Geometry: final body of the model. Coordinates: model frame, mm. A direction names the side the tool comes from. Round coordinates to 2 decimals unless told otherwise and drop trailing zeros. Order: outer loops, then holes, each group sorted by start corner. A loop starts at its lowest first (then second) coordinate and runs counter-clockwise, first axis right, second up. Notation, with made-up numbers: M 83.5,80 L 113.5,80 A19 cw 113.5,113 Z; hole C 60.5,-37 d7. An arc over 180 degrees is marked long. Put each result on its own line as item: value. Start each with the question number.
1) Section A-A, the plane x = -5. Return loops of the section in (y, z) (3 decimals).
2) Section D-D, the plane x = 9.5. Return loops of the section in (y, z), then the cut area to 3 significant figures.
3) Access query for faces 1 (the flat face through (6.25, 0, 0)), 2 (the flat face through (-25, 0, 0)). Directions: +Z, -Z, +X, -X, +Y, -Y. A direction counts if a zero-diameter tool reaches every point of the face in a straight line with its end or side. Return the directions, or none.
4) First-contact query: P1, Ø3, axis at x = -21.92, z = -21.92, coming from the +Y side. Flat tip, straight axial feed; report the tip coordinate or a pass-through.
5) Section C-C, the plane y = -0.85. Return loops of the section in (x, z) (3 decimals), then the cut area to 3 significant figures.
6) Draft query along X for faces 3 (the flat face through (0, 0, -25)), 4 (the cylindrical face through (23.797, 0.02, 23.859)), 5 (the flat face through (0, 0, -11.625)), 6 (the flat face through (-6.25, 0, 0)). Return one class per face: pulls with the +X half, pulls with the -X half, needs draft (parallel to the pull), parting line crosses it, or undercut.
7) Section B-B, the plane z = 0. Return loops of the section in (x, y).
8) Material intervals for probe 1 along X at (y, z) = (0.6, 0); probe 2 along Z at (x, y) = (2, -0.3) (3 decimals); probe 3 along X at (y, z) = (0.4, -10.5), sorted ascending. Write a range as [from, to].
Autodesk Inventor part; units mm, degrees
ref_plane "YZ Plane" through (0, 0, 0) normal (1, 0, 0) x (0, 1, 0)
ref_plane "XZ Plane" through (0, 0, 0) normal (0, 1, 0) x (-1, 0, 0)
ref_plane "XY Plane" through (0, 0, 0) normal (0, 0, 1) x (1, 0, 0)
sketch "Sketch1" plane through (0, 0, 0) normal (0, 1, 0) x (-1, 0, 0)
  line L0 (-25, 25) -> (25, 25)
  line L1 (25, 25) -> (25, -25)
  line L2 (25, -25) -> (-25, -25)
  line L3 (-25, -25) -> (-25, 25)
  line L4 (-25, 25) -> (25, -25) construction
  line L5 (25, 25) -> (-25, -25) construction
  point P0 (0, 0)
  dimension "d0" = 50
extrude "Extrusion1" add sketch "Sketch1" along normal mid plane 2.8
sketch "Sketch2" plane through (0, 1.4, 0) normal (0, 1, 0) x (1, 0, 0)
  line L0 (-6.25, -11.625) -> (6.25, -11.625)
  line L1 (6.25, -11.625) -> (6.25, 11.625)
  line L2 (6.25, 11.625) -> (-6.25, 11.625)
  line L3 (-6.25, 11.625) -> (-6.25, -11.625)
  line L4 (-6.25, -11.625) -> (6.25, 11.625) construction
  line L5 (6.25, -11.625) -> (-6.25, 11.625) construction
  point P0 (0, 0)
  dimension "d3" = 12.5
  dimension "d4" = 23.25
extrude "Extrusion2" cut sketch "Sketch2" against normal through all
sketch "Sketch3" plane through (0, 1.4, 0) normal (0, 1, 0) x (1, 0, 0)
  line L0 (6.25, 11.625) -> (6.25, -11.625) construction
  line L1 (6.25, -11.625) -> (-6.25, -11.625) construction
  line L2 (-6.25, -11.625) -> (-6.25, 11.625) construction
  line L3 (-6.25, 11.625) -> (6.25, 11.625) construction
  line L4 (-25, -25) -> (25, -25) construction
  line L5 (25, -25) -> (25, 25) construction
  line L6 (25, 25) -> (-25, 25) construction
  line L7 (-25, 25) -> (-25, -25) construction
  line L8 (-21.9203, 21.9203) -> (21.9203, 21.9203)
  line L9 (21.9203, 21.9203) -> (21.9203, -21.9203)
  line L10 (21.9203, -21.9203) -> (-21.9203, -21.9203)
  line L11 (-21.9203, -21.9203) -> (-21.9203, 21.9203)
  line L12 (-9.5, 14.875) -> (-9.5, -14.875)
  line L13 (-9.5, -14.875) -> (9.5, -14.875)
  line L14 (9.5, -14.875) -> (9.5, 14.875)
  line L15 (9.5, 14.875) -> (-9.5, 14.875)
  point P0 (0, 0)
  point P1 (-9.5, 0)
  point P2 (9.5, 0)
  dimension "d7" = 62
  dimension "d8" = 19
hole "Hole1" at (-21.9203, 1.4, -21.9203) at (21.9203, 1.4, -21.9203) at (21.9203, 1.4, 21.9203) at (-21.9203, 1.4, 21.9203) at (-9.5, 1.4, 0) at (9.5, 1.4, 0) direction (0, -1, 0) diameter 2.5 end through all
fillet "Fillet1" radius 4 4 edges at (-25, 0, -25) (25, 0, -25) (25, 0, 25) (-25, 0, 25)
Result sheet:
1. outline: M -1.4,-25 L 1.4,-25 L 1.4,-11.625 L -1.4,-11.625 Z; M -1.4,11.625 L 1.4,11.625 L 1.4,25 L -1.4,25 Z
2. outline: M -1.4,-25 L 1.4,-25 L 1.4,-1.25 L -1.4,-1.25 Z; M -1.4,1.25 L 1.4,1.25 L 1.4,25 L -1.4,25 Z
2. area: 133 mm2
3. face 1: +Y, -Y
3. face 2: +Z, -Z, -X, +Y, -Y
4. P1: stops at y = 1.4
5. outline: M -25,-21 A4 ccw -21,-25 L 21,-25 A4 ccw 25,-21 L 25,21 A4 ccw 21,25 L -21,25 A4 ccw -25,21 Z; hole C -21.92,-21.92 d2.5; hole C -21.92,21.92 d2.5; hole C -9.5,0 d2.5; hole M -6.25,-11.625 L 6.25,-11.625 L 6.25,11.625 L -6.25,11.625 Z; hole C 9.5,0 d2.5; hole C 21.92,-21.92 d2.5; hole C 21.92,21.92 d2.5
5. area: 2,170 mm2
6. face 3: needs draft
6. face 4: pulls with the +X half
6. face 5: undercut
6. face 6: undercut
7. outline: M -25,-1.4 L -10.75,-1.4 L -10.75,1.4 L -25,1.4 Z; M -8.25,-1.4 L -6.25,-1.4 L -6.25,1.4 L -8.25,1.4 Z; M 6.25,-1.4 L 8.25,-1.4 L 8.25,1.4 L 6.25,1.4 Z; M 10.75,-1.4 L 25,-1.4 L 25,1.4 L 10.75,1.4 Z
8. probe 1: x = [-25, -10.75], [-8.25, -6.25], [6.25, 8.25], [10.75, 25]
8. probe 2: z = [-25, -11.625], [11.625, 25]
8. probe 3: x = [-25, -6.25], [6.25, 25]
